from build123d import *

# Parameters (mm, degrees)
SKETCH1_R                     = 7.5
SKETCH1_R_2                   = 4.2
BOSS_EXTRUDE1_DEPTH           = 47
SKETCH2_R                     = 11.2
CUT_EXTRUDE1_DEPTH            = 7
SKETCH3_R                     = 2.25
SKETCH3_R_2                   = 12
CUT_EXTRUDE2_DEPTH            = 15
CUT_EXTRUDE3_DEPTH            = 85.391942743
CUT_EXTRUDE4_DEPTH            = 20
SKETCH7_R                     = 2.6
CUT_EXTRUDE5_DEPTH            = 10
CHAMFER2_SIZE                 = 1
SKETCH9_W                     = 25
SKETCH9_H                     = 47
BOSS_EXTRUDE2_DEPTH           = 7
BOSS_EXTRUDE2_2_DEPTH         = 7
SKETCH10_W                    = 2.9
SKETCH10_H                    = 7
M5_CLEARANCE_HOLE1_AT_2_COUNT = 2
M5_CLEARANCE_HOLE1_AT_2_PITCH = 25
M5_CLEARANCE_HOLE1_AT_3_COUNT = 2
M5_CLEARANCE_HOLE1_AT_3_PITCH = 114.756263446
M5_CLEARANCE_HOLE1_AT_4_COUNT = 2
M5_CLEARANCE_HOLE1_AT_4_PITCH = 112
BOSS_EXTRUDE3_DEPTH           = 47
FILLET1_R                     = 5


with BuildPart() as part:
    # Sketch1 → Boss-Extrude1 (new body)
    with BuildSketch(Plane.XY):
        Polygon((-30, -25), (-30, 22), (22, 22), (52, 8), (52, -25), align=None)
        Circle(SKETCH1_R, mode=Mode.SUBTRACT)
        with Locations((40, 0)):
            Circle(SKETCH1_R_2, mode=Mode.SUBTRACT)
    extrude(amount=BOSS_EXTRUDE1_DEPTH)

    # Sketch2 → Cut-Extrude1 (cut)
    with BuildSketch(Plane.XY.offset(47)):
        Circle(SKETCH2_R)
    extrude(amount=-CUT_EXTRUDE1_DEPTH, mode=Mode.SUBTRACT)

    # Sketch3 → Cut-Extrude2 (cut)
    with BuildSketch(Plane(origin=(0, 0, 0), x_dir=(-1, 0, 0), z_dir=(0, 0, -1))):
        with Locations((-15.5, 15.5)):
            Circle(SKETCH3_R)
        with Locations((-15.5, -15.5)):
            Circle(SKETCH3_R)
        with Locations((15.5, -15.5)):
            Circle(SKETCH3_R)
        with Locations((15.5, 15.5)):
            Circle(SKETCH3_R)
        Circle(SKETCH3_R_2)
    extrude(amount=-CUT_EXTRUDE2_DEPTH, mode=Mode.SUBTRACT)

    # Sketch4 → Cut-Extrude3 (cut, through all)
    with BuildSketch(Plane(origin=(0, 22, 0), x_dir=(1, 0, 0), z_dir=(0, 1, 0))):
        with BuildLine():
            Line((-19, -7), (41, -7))
            ThreePointArc((41, -7), (44.535533906, -8.464466094), (46, -12))
            Line((46, -12), (46, -32))
            ThreePointArc((46, -32), (44.535533906, -35.535533906), (41, -37))
            Line((41, -37), (-19, -37))
            ThreePointArc((-19, -37), (-22.535533906, -35.535533906), (-24, -32))
            Line((-24, -32), (-24, -12))
            ThreePointArc((-24, -12), (-22.535533906, -8.464466094), (-19, -7))
        make_face()
    extrude(amount=-CUT_EXTRUDE3_DEPTH, mode=Mode.SUBTRACT)

    # Sketch6 → Cut-Extrude4 (cut)
    with BuildSketch(Plane.XY.offset(47)):
        with BuildLine():
            Line((-19.5, -12), (-19.5, -18))
            ThreePointArc((-19.5, -18), (-15.5, -22), (-11.5, -18))
            Line((-11.5, -18), (-11.5, -12))
            ThreePointArc((-11.5, -12), (-15.5, -8), (-19.5, -12))
        make_face()
        with BuildLine():
            Line((11.5, -12), (11.5, -18))
            ThreePointArc((11.5, -18), (15.5, -22), (19.5, -18))
            Line((19.5, -18), (19.5, -12))
            ThreePointArc((19.5, -12), (15.5, -8), (11.5, -12))
        make_face()
    extrude(amount=-CUT_EXTRUDE4_DEPTH, mode=Mode.SUBTRACT)

    # Sketch7 → Cut-Extrude5 (cut)
    with BuildSketch(Plane(origin=(52, 0, 0), x_dir=(0, 0, -1), z_dir=(1, 0, 0))):
        with Locations(Location((-42, 0, 0), (0, 0, 90))):
            Circle(SKETCH7_R)
    extrude(amount=-CUT_EXTRUDE5_DEPTH, mode=Mode.SUBTRACT)

    # Chamfer2
    chamfer2_edges = [part.edges().sort_by_distance(p)[0] for p in [
        (52, -2.6, 42),
    ]]
    chamfer(chamfer2_edges, length=CHAMFER2_SIZE)



with BuildPart() as body_2:
    # Sketch9 → Boss-Extrude2 (new body)
    with BuildSketch(Plane.XZ.offset(25)):
        with Locations((-42.5, 23.5)):
            Rectangle(SKETCH9_W, SKETCH9_H)
    extrude(amount=-BOSS_EXTRUDE2_DEPTH)

    # Sketch10 → M5 Clearance Hole1 (revolve, cut)
    with BuildSketch(Plane(origin=(-45, -18, 36), x_dir=(0, 0, 1), z_dir=(1, 0, 0))):
        with Locations((1.45, 3.5)):
            Rectangle(SKETCH10_W, SKETCH10_H)
    m5_clearance_hole1 = revolve(axis=Axis((-45, -11.65, 36), (0, -1, 0)), mode=Mode.SUBTRACT)

    # M5 Clearance Hole1 at 2: M5 Clearance Hole1 ×2
    with Locations(*[(0, 0, -i * M5_CLEARANCE_HOLE1_AT_2_PITCH) for i in range(1, M5_CLEARANCE_HOLE1_AT_2_COUNT)]):
        add(m5_clearance_hole1, mode=Mode.SUBTRACT)


with BuildPart() as body_3:
    # Sketch9 → Boss-Extrude2 2 (new body)
    with BuildSketch(Plane.XZ.offset(25)):
        with Locations((64.5, 23.5)):
            Rectangle(SKETCH9_W, SKETCH9_H)
    extrude(amount=-BOSS_EXTRUDE2_2_DEPTH)

    # M5 Clearance Hole1 at 3: M5 Clearance Hole1 ×2
    with Locations(*[Vector(0.9759815859905214, 0, -0.21785303258717012) * (i * M5_CLEARANCE_HOLE1_AT_3_PITCH) for i in range(1, M5_CLEARANCE_HOLE1_AT_3_COUNT)]):
        add(m5_clearance_hole1, mode=Mode.SUBTRACT)

    # M5 Clearance Hole1 at 4: M5 Clearance Hole1 ×2
    with Locations(*[(i * M5_CLEARANCE_HOLE1_AT_4_PITCH, 0, 0) for i in range(1, M5_CLEARANCE_HOLE1_AT_4_COUNT)]):
        add(m5_clearance_hole1, mode=Mode.SUBTRACT)


with BuildPart() as part_1:
    add(part.part)

    add(body_2.part)  # Boss-Extrude3 merges body 2

    add(body_3.part)  # Boss-Extrude3 merges body 3
    # Sketch13 → Boss-Extrude3 (add)
    with BuildSketch(Plane(origin=(0, 0, 0), x_dir=(-1, 0, 0), z_dir=(0, 0, -1))):
        Polygon((-52, -18), (-58, -18), (-52, -12), align=None)
        Polygon((30, -18), (30, -12), (36, -18), align=None)
    extrude(amount=-BOSS_EXTRUDE3_DEPTH)

    # Fillet1
    fillet1_edges = [part_1.edges().sort_by_distance(p)[0] for p in [
        (-55, -21.5, 47),
        (-55, -21.5, 0),
        (77, -21.5, 0),
        (77, -21.5, 47),
    ]]
    fillet(fillet1_edges, radius=FILLET1_R)


solid = part_1.part
The model under review builds one solid part; all positions refer to its coordinate system, in mm. A direction names the side the tool comes from. Give positions to 0.01 mm unless a question says otherwise; leave off trailing zeros. Order: outer loops, then holes, each group sorted by start corner. A loop starts at its lowest first (then second) coordinate and runs counter-clockwise, first axis right, second up. Notation, with made-up numbers: (-12, -5) -> (30, -5) arc R20 ccw to (30, 1) -> close; hole circle Ø10 at (80.25, 36). An arc over 180 degrees is marked (long way). Write item = value, one per line. Start each with the question number.
(1) For pin 1 Ø4 at (y, z) = (-9, 12.5) entering from +X; pin 2 Ø6 at (y, z) = (0, 42) entering from +X; pin 3 Ø6.5 at (x, y) = (-4.5, -4) entering from +Z, all flat-tipped, find the tip position at first contact; note any pin that passes through.
(2) Take a section at C-C (x = -15.5). Write out the cut boundary in (y, z), plus the area to 3 significant figures.
(3) Take a section at D-D (x = 30.5). Write out the cut boundary in (y, z).
(4) Take a section at A-A (z = 25). Write out the cut boundary in (x, y).
(5) Tool access review of faces 4 (the cylindrical face through (11.99, 0.53, 3.45)), 5 (the flat face through (11.5, -15, 42)), 6 (the flat face through (-46, -18, 24)): name each direction out of +Z, -Z, +X, -X, +Y, -Y from which nothing blocks a thin tool from reaching the whole face with its end or side.
(6) Take a section at B-B (x = -45). Write out the cut boundary in (y, z).
(7) Draft analysis for pull direction Z (two halves, no side actions). For faces 1 (the cylindrical face through (15.6, -8, 42.1)), 2 (the cylindrical face through (45, -6, 35)), 3 (the cylindrical face through (-53, -21, 46)), state which applies: +Z half, -Z half, draft (parallel to the pull), parting line (faces both ways), or undercut.
(8) For L1, parallel to X at y = 0, z = 38.3; L2, parallel to Z at x = -45, y = -22; L3, parallel to Z at x = 35, y = -7, list the stretches that pass through material, from the lowest coordinate up. Write a range as from..to.
Returned:
q1.pin_1 = 52
q1.pin_2 = 51.4
q1.pin_3 = 40
q2.outline = (-25, 0) -> (-17.75, 0) -> (-17.75, 7) -> (-25, 7) -> close; (-25, 37) -> (-22, 37) -> (-22, 47) -> (-25, 47) -> close; (-13.25, 0) -> (13.25, 0) -> (13.25, 7) -> (-13.25, 7) -> close; (-8, 37) -> (22, 37) -> (22, 47) -> (-8, 47) -> close; (17.75, 0) -> (22, 0) -> (22, 7) -> (17.75, 7) -> close
q2.area = 596 mm²
q3.outline = (-25, 0) -> (18.03, 0) -> (18.03, 7) -> (-25, 7) -> close; (-25, 37) -> (18.03, 37) -> (18.03, 47) -> (-25, 47) -> close
q4.outline = (-55, -25) -> (-24, -25) -> (-24, 22) -> (-30, 22) -> (-30, -12) -> (-36, -18) -> (-55, -18) -> close; (46, -25) -> (77, -25) -> (77, -18) -> (58, -18) -> (52, -12) -> (52, 8) -> (46, 10.8) -> close
q5.face_4 = -Z
q5.face_5 = +Z
q5.face_6 = +Z, -Z, -X, +Y
q6.outline = (-25, 0) -> (-18, 0) -> (-18, 8.1) -> (-25, 8.1) -> close; (-25, 13.9) -> (-18, 13.9) -> (-18, 33.1) -> (-25, 33.1) -> close; (-25, 38.9) -> (-18, 38.9) -> (-18, 47) -> (-25, 47) -> close
q7.face_1 = draft
q7.face_2 = undercut
q7.face_3 = +Z half
q8.L1 = -30..-7.5, 7.5..35.8, 44.2..52
q8.L2 = 0..8.1, 13.9..33.1, 38.9..47
q8.L3 = 0..7, 37..47
